The listing builds one solid part. Answer for the finished solid, in the listing's coordinates (mm). A direction names the side the tool comes from. Give positions to 0.01 mm unless a question says otherwise; leave off trailing zeros. Write each loop counter-clockwise with the first axis right and the second up, starting at its lowest first coordinate (ties: lowest second). Pieces come first, ordered by that corner, then holes. Notation, with made-up numbers: (33.5, 0.25) - (51.5, 0.25) arc R28 ccw to (51.5, 30.25) - close; hole circle Ø4 at (-3, 24.25). An arc over 180 degrees is marked (long way). Return JSON: item names as keys, results as strings.
from build123d import *

# Parameters (mm, degrees)
ODEBRAT_VYSUNUT_M1_REACH = 22
SKICA2_R                 = 5
P_IDAT_START             = -7.597862
P_IDAT_VYSUNUT_M1_DEPTH  = 17.597862
KRUHOV_POLE1_COUNT       = 5


with BuildPart() as part:
    # Skica1 → Rotovat1 (revolve)
    with BuildSketch(Plane.XY):
        with BuildLine():
            Line((0, 0), (0, 20))
            Line((0, 20), (14, 20))
            ThreePointArc((14, 20), (32.579084411, 17.662353543), (50, 10.795136598))
            Line((50, 10.795136598), (50, 0))
            Line((50, 0), (0, 0))
        make_face()
    revolve(axis=Axis((0, 0, 0), (0, 1, 0)))

    # Skica2 → Odebrat vysunutím1 (cut, up to next)
    with BuildSketch(Plane(origin=(0, 20, 0), x_dir=(1, 0, 0), z_dir=(0, 1, 0)), mode=Mode.PRIVATE) as odebrat_vysunut_m1_sk1:
        Circle(SKICA2_R)
    odebrat_vysunut_m1_tool1 = extrude(odebrat_vysunut_m1_sk1.sketch, amount=-ODEBRAT_VYSUNUT_M1_REACH, mode=Mode.PRIVATE) & part.part
    add(odebrat_vysunut_m1_tool1.solids().sort_by_distance((0, 20, 0))[0], mode=Mode.SUBTRACT)

    # Skica3 → Přidat vysunutím1 (add)
    with BuildSketch(Plane(origin=(0, 20, 0), x_dir=(1, 0, 0), z_dir=(0, 1, 0)).offset(P_IDAT_START)):
        with BuildLine():
            ThreePointArc((5.542949714, 44.202455598), (4.287230231, 46.631857241), (1.78118303, 45.537073612))
            ThreePointArc((1.78118303, 45.537073612), (-2.260445719, 32.522428192), (-3.499658814, 18.951130934))
            ThreePointArc((-3.499658814, 18.951130934), (0.216435534, 15.506698459), (3.478925663, 19.383505191))
            ThreePointArc((3.478925663, 19.383505191), (3.31115986, 31.892757792), (5.542949714, 44.202455598))
        make_face()
    p_idat_vysunut_m1 = extrude(amount=P_IDAT_VYSUNUT_M1_DEPTH)

    # Kruhové pole1: Přidat vysunutím1 ×5 about axis
    kruhov_pole1_axis = Axis((0, 0, 0), (0, 1, 0))
    for i in range(1, KRUHOV_POLE1_COUNT):
        add(p_idat_vysunut_m1.rotate(kruhov_pole1_axis, i * 360 / KRUHOV_POLE1_COUNT))


solid = part.part
Item 1: Flat-ended cylindrical pins translate along their axes: P1, Ø3, axis at x = -3.5, z = 26.5, coming from the +Y side; P2, Ø1.5, axis at x = 5.5, y = 6, coming from the +Z side; P3, Ø10, axis at x = 20, y = 8, coming from the -Z side; P4, Ø4, axis at x = -30.5, z = -32.5, coming from the -Y side. Find the tip coordinate at first contact, or state that the pin passes through.
Answer below:
{"P1": "stops at y = 19.15", "P2": "stops at z = 49.77", "P3": "stops at z = -47.7", "P4": "stops at y = 0"}
Item 2: For faces 1 (the face through (9.001, 24.82, 12.623)), 2 (the face through (-21.31, 23.47, 23.72)), 3 (the face through (15.976, 23.466, 27.598)), 4 (the face through (-1, 0, 10)), 5 (the face through (45.673, 21.078, -10.291)), determine the directions among +Z, -Z, +X, -X, +Y, -Y from which every point of the face is accessible in a straight line to the end or side of a thin tool.
Answer below:
{"face 1": "+Y", "face 2": "-X, +Y", "face 3": "+Z, +Y", "face 4": "+Z, -Z, +X, -X, -Y", "face 5": "+X, +Y"}
Item 3: Consider L1, parallel to Z at x = 0, y = 9; L2, parallel to Z at x = 0, y = 11. Determine where each line is inside the solid, lowest interval first.
Answer below:
{"L1": "z = -50 to -5, 5 to 50", "L2": "z = -49.62 to -5, 5 to 49.62"}
Item 4: A cutting plane is placed at A-A on y = 6.5. Determine the outline of the cut face in (x, z), then the cut area to 3 significant figures.
Answer below:
{"outline": "circle Ø100 at (0, 0); hole circle Ø10 at (0, 0)", "area": "7,780 mm²"}
Item 5: The mould has two halves that part along Z. Classify faces 6 (the face through (-17.43, 23.28, 27.77)), 7 (the face through (1, 30, -28)), 8 (the face through (31.184, 23.466, -6.666)): +Z half, -Z half, draft (parallel to the pull), parting line (faces both ways), or undercut.
Answer below:
{"face 6": "+Z half", "face 7": "draft", "face 8": "undercut"}
